Part print with two shaded views. Sizes in mm from the minimum x, y, z corner. A direction names the side the tool comes from. Coordinates: 2 decimals unless noted, no trailing zeros. Loops run counter-clockwise (first coordinate to the right, second up) from the corner with the lowest first, then second, coordinate; pieces in that order, holes last.
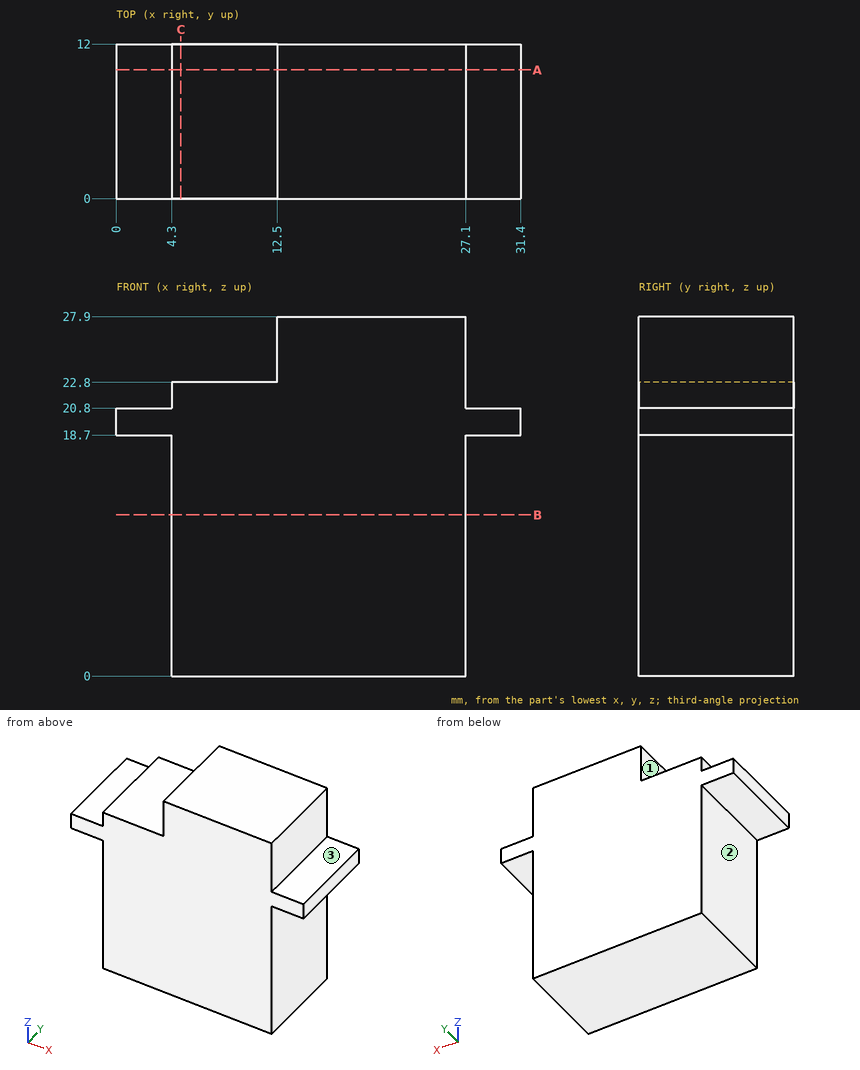
Q1. Slice it at C-C (x = 5). List the corners of the cut face in (y, z), and give its area (3 significant figures).
Answers:
outline: (0, 0) - (12, 0) - (12, 22.8) - (0, 22.8) - close
area: 274 mm2
Q2. Drill centre lines: line 1 (X direction, y = 4, z = 13.5); line 2 (X direction, y = 6.75, z = 23.5); line 3 (Z direction, x = 2.5, y = 6.5). Where is each one in solid material? Low to high.
Answers:
line 1: x = 4.3 to 27.1
line 2: x = 12.5 to 27.1
line 3: z = 18.7 to 20.8
Q3. Flat gauge pins, fed straight in: P1, Ø4.5, axis at x = 30, y = 4, coming from the -Z side; P2, Ø6, axis at y = 4.5, z = 15, coming from the +X side; P3, Ø3.5, axis at x = 2.5, y = 8, coming from the +Z side. Where does each tip first touch, or does it go through?
Answers:
P1: stops at z = 18.7
P2: stops at x = 27.1
P3: stops at z = 20.8
Q4. Slice it at A-A (y = 10). List the corners of the cut face in (x, z).
Answers:
outline: (0, 18.7) - (4.3, 18.7) - (4.3, 0) - (27.1, 0) - (27.1, 18.7) - (31.4, 18.7) - (31.4, 20.8) - (27.1, 20.8) - (27.1, 27.9) - (12.5, 27.9) - (12.5, 22.8) - (4.3, 22.8) - (4.3, 20.8) - (0, 20.8) - close
Q5. Slice it at B-B (z = 12.5). List the corners of the cut face in (x, y), and give its area (3 significant figures).
Answers:
outline: (4.3, 0) - (27.1, 0) - (27.1, 12) - (4.3, 12) - close
area: 274 mm2
Q6. Which spindle directions (+Z, -Z, +X, -X, +Y, -Y) get a long thin tool onto all of the face, cutting with end or side? Do the marked faces 1, 2 and 3. Say none if no direction does.
Answers:
face 1: +Z, -X, +Y, -Y
face 2: -Z, -X, +Y, -Y
face 3: +Z, +X, +Y, -Y
